```python
from build123d import *

# Parameters (mm, degrees)
SKETCH1_R           = 1.5
SKETCH1_R_2         = 1.65
BOSS_EXTRUDE1_DEPTH = 5.842
FILLET2_R           = 11
SKETCH2_R           = 0.5
CUT_EXTRUDE1_DEPTH  = 73.079185373


with BuildPart() as part:
    # Sketch1 → Boss-Extrude1 (new body)
    with BuildSketch(Plane.XY):
        with BuildLine():
            Line((22.325000054, -37.323), (22.325000054, 28.495993037))
            Line((22.325000054, 28.495993037), (22.325000054, 45.631506359))
            ThreePointArc((22.325000054, 45.631506359), (0, -50.8), (-22.325000054, 45.631506359))
            Line((-22.325000054, 45.631506359), (-22.325000054, 28.495993037))
            Line((-22.325000054, 28.495993037), (-22.325000054, -37.323))
            Line((-22.325000054, -37.323), (22.325000054, -37.323))
        make_face()
        with Locations((-45.72, 0)):
            Circle(SKETCH1_R, mode=Mode.SUBTRACT)
        with Locations((45.72, 0)):
            Circle(SKETCH1_R, mode=Mode.SUBTRACT)
        with Locations((0, -45.72)):
            Circle(SKETCH1_R, mode=Mode.SUBTRACT)
        with Locations((39.594681461, 22.86)):
            Circle(SKETCH1_R_2, mode=Mode.SUBTRACT)
        with Locations((39.594681461, -22.86)):
            Circle(SKETCH1_R_2, mode=Mode.SUBTRACT)
        with Locations((-39.594681461, -22.86)):
            Circle(SKETCH1_R_2, mode=Mode.SUBTRACT)
        with Locations((-39.594681461, 22.86)):
            Circle(SKETCH1_R_2, mode=Mode.SUBTRACT)
    extrude(amount=BOSS_EXTRUDE1_DEPTH)

    # Fillet2
    fillet2_edges = [part.edges().sort_by_distance(p)[0] for p in [
        (22.325000054, 45.631506359, 2.921),
        (-22.325000054, 45.631506359, 2.921),
    ]]
    fillet(fillet2_edges, radius=FILLET2_R)

    # Sketch2 → Cut-Extrude1 (cut, through all)
    with BuildSketch(Plane.XY.offset(5.842)):
        with Locations((-22.325000054, -37.323)):
            Circle(SKETCH2_R)
        with Locations((22.325000054, -37.323)):
            Circle(SKETCH2_R)
    extrude(amount=-CUT_EXTRUDE1_DEPTH, mode=Mode.SUBTRACT)


solid = part.part
```
Here's how the part is built. I have some questions about the finished solid (model axes, mm). A direction names the side the tool comes from. Round coordinates to 2 decimals unless told otherwise and drop trailing zeros. Write each loop counter-clockwise with the first axis right and the second up, starting at its lowest first coordinate (ties: lowest second). Pieces come first, ordered by that corner, then holes.
Q1. If we mould it in two halves opening along Y, with no side actions, what happens to faces 1 (the cylindrical face through (-44.29, 0.45, 2.88)), 2 (the cylindrical face through (-0.195, -44.233, 2.88)), 3 (the flat face through (-22.325, -7, 3)), 4 (the cylindrical face through (-30.38, 32.36, 2.96))? For each: +Y half, -Y half, draft (parallel to the pull), parting line (faces both ways), or undercut.
Q2. If we section it at D-D on y = -45.72: Write out the boundary of the cut face in (x, z), plus the area to 3 significant figures.
Q3. If we section it at C-C on z = 2: Write out the boundary of the cut face in (x, y) (3 decimals), plus the area to 3 significant figures.
Q4. Will these pins go through, and if not, where does the flat tip stop? P1, Ø3, axis at x = 6.5, z = 1.5, coming from the +Y side; P2, Ø1, axis at x = 2.5, z = 2.5, coming from the -Y side; P3, Ø1, axis at x = 15, z = 2, coming from the -Y side.
Q5. If we section it at A-A on x = 0: Write out the boundary of the cut face in (y, z).
Q6. Which directions (+Z, -Z, +X, -X, +Y, -Y) give clear straight access to the entire face, cutting with the end or side of a thin tool? Please do faces 5 (the flat face through (0, -37.323, 3)), 6 (the flat face through (23, -8, 0)).
Q7. Please list where these lines run through material, in increasing order: probe 1 along Y at (x, z) = (0, 3.95); probe 2 along Y at (x, z) = (-45.72, 1.6); probe 3 along X at (y, z) = (-23, 3.05) (3 decimals).
Q8. If we section it at B-B on y = 0: Write out the boundary of the cut face in (x, z) (3 decimals), plus the area to 3 significant figures.
Answer below:
1. face 1: undercut
1. face 2: undercut
1. face 3: draft
1. face 4: +Y half
2. outline: (-22.14, 0) - (-1.5, 0) - (-1.5, 5.84) - (-22.14, 5.84) - close; (1.5, 0) - (22.14, 0) - (22.14, 5.84) - (1.5, 5.84) - close
2. area: 241 mm2
3. outline: (-42.535, 27.774) arc R50.8 ccw (long way) to (42.535, 27.774) arc R11 ccw to (22.325, 21.76) - (22.325, -36.823) arc R0.5 cw (long way) to (21.825, -37.323) - (-21.825, -37.323) arc R0.5 cw (long way) to (-22.325, -36.823) - (-22.325, 21.76) arc R11 ccw to start; hole circle Ø3 at (-45.72, 0); hole circle Ø3.3 at (-39.595, -22.86); hole circle Ø3.3 at (-39.595, 22.86); hole circle Ø3 at (0, -45.72); hole circle Ø3.3 at (39.595, -22.86); hole circle Ø3.3 at (39.595, 22.86); hole circle Ø3 at (45.72, 0)
3. area: 3,890 mm2
4. P1: stops at y = -37.32
4. P2: stops at y = -50.76
4. P3: stops at y = -48.69
5. outline: (-50.8, 0) - (-47.22, 0) - (-47.22, 5.84) - (-50.8, 5.84) - close; (-44.22, 0) - (-37.32, 0) - (-37.32, 5.84) - (-44.22, 5.84) - close
6. face 5: +Z, -Z, +Y
6. face 6: -Z, +X, -X, +Y, -Y
7. probe 1: y = -50.8 to -47.22, -44.22 to -37.32
7. probe 2: y = -22.14 to -1.5, 1.5 to 22.14
7. probe 3: x = -45.295 to -41.239, -37.951 to -22.325, 22.325 to 37.951, 41.239 to 45.295
8. outline: (-50.8, 0) - (-47.22, 0) - (-47.22, 5.842) - (-50.8, 5.842) - close; (-44.22, 0) - (-22.325, 0) - (-22.325, 5.842) - (-44.22, 5.842) - close; (22.325, 0) - (44.22, 0) - (44.22, 5.842) - (22.325, 5.842) - close; (47.22, 0) - (50.8, 0) - (50.8, 5.842) - (47.22, 5.842) - close
8. area: 298 mm2
